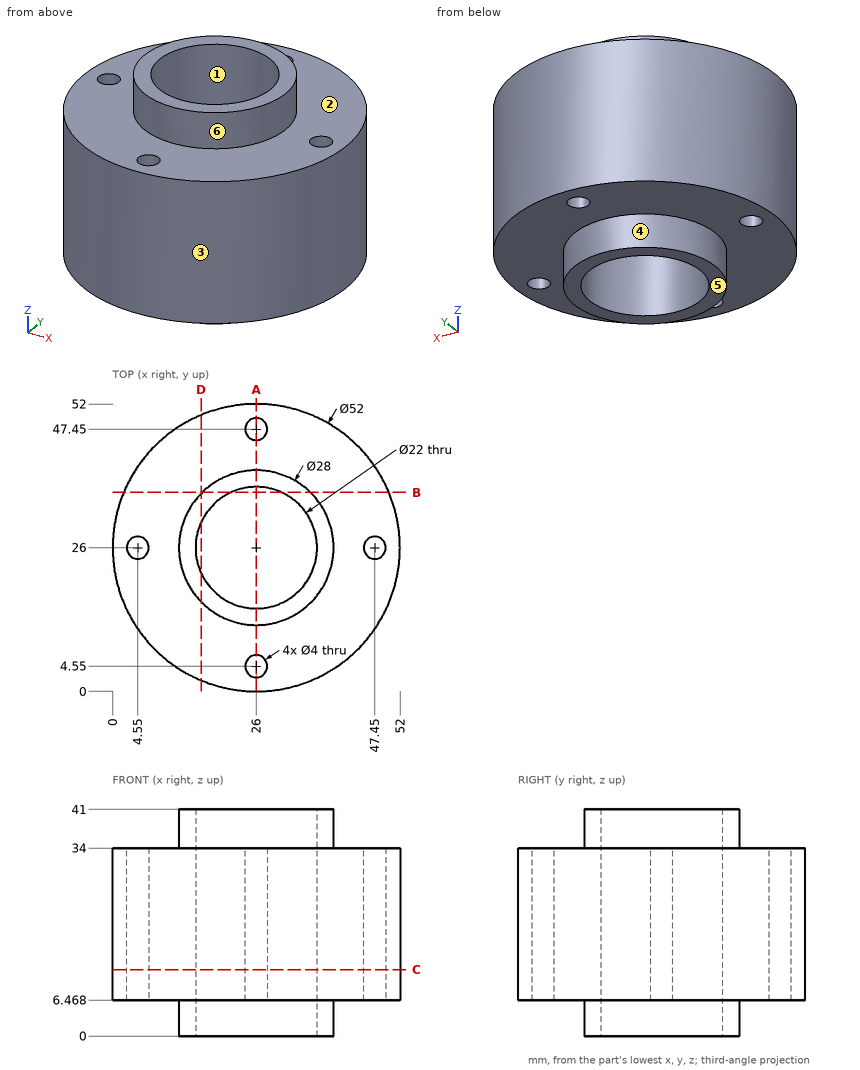
Study the drawing (mm; zero at the part's minimum x, y, z) and answer. A direction names the side the tool comes from. Give positions to 0.01 mm unless a question says otherwise; leave off trailing zeros. Order: outer loops, then holes, each group sorted by start corner. A loop starts at its lowest first (then second) coordinate and runs counter-clockwise, first axis right, second up.
1. Straight lines are drawn through the part: L1, parallel to Y at x = 26, z = 22; L2, parallel to Y at x = 26.5, z = 36; L3, parallel to Z at x = 13.5, y = 15.5. For each, find the intervals that lie inside material, in ascending order.
Result sheet:
L1: y = 0 to 2.55, 6.55 to 15, 37 to 45.45, 49.45 to 52
L2: y = 12.01 to 15.01, 36.99 to 39.99
L3: z = 6.47 to 34
2. Each of these flat-tipped pins is pushed along its axis until it touches: P1, Ø1.5, axis at x = 18, y = 6, coming from the -Z side; P2, Ø1.5, axis at y = 38, z = 14, coming from the +X side; P3, Ø1.5, axis at x = 16, y = 25, coming from the -Z side; P4, Ø5, axis at y = 26.5, z = 5, coming from the -X side. Where does it stop, or does it pass through?
Result sheet:
P1: stops at z = 6.47
P2: stops at x = 49.44
P3: passes through
P4: stops at x = 0
3. Section B-B, the plane y = 36 is taken. Determine the outline of the cut face in (x, z).
Result sheet:
outline: (2, 6.47) - (16.2, 6.47) - (16.2, 0) - (21.42, 0) - (21.42, 41) - (16.2, 41) - (16.2, 34) - (2, 34) - close; (30.58, 0) - (35.8, 0) - (35.8, 6.47) - (50, 6.47) - (50, 34) - (35.8, 34) - (35.8, 41) - (30.58, 41) - close
4. Section A-A, the plane x = 26 is taken. Determine the outline of the cut face in (y, z).
Result sheet:
outline: (0, 6.47) - (2.55, 6.47) - (2.55, 34) - (0, 34) - close; (6.55, 6.47) - (12, 6.47) - (12, 0) - (15, 0) - (15, 41) - (12, 41) - (12, 34) - (6.55, 34) - close; (37, 0) - (40, 0) - (40, 6.47) - (45.45, 6.47) - (45.45, 34) - (40, 34) - (40, 41) - (37, 41) - close; (49.45, 6.47) - (52, 6.47) - (52, 34) - (49.45, 34) - close
5. The mould has two halves that part along X. Classify the marked faces 1, 2 and 3: released by +X, released by -X, zero draft, split by the parting line, or undercut.
Result sheet:
face 1: undercut
face 2: zero draft
face 3: split by the parting line
6. For the marked faces 4, 5 and 6, determine the directions among +Z, -Z, +X, -X, +Y, -Y from which every point of the face is accessible in a straight line to the end or side of a thin tool.
Result sheet:
face 4: -Z
face 5: -Z, +X, -X, +Y, -Y
face 6: +Z
7. Section C-C, the plane z = 12 is taken. Determine the outline of the cut face in (x, y), and give its area (3 significant figures).
Result sheet:
outline: circle Ø52 at (26, 26); hole circle Ø4 at (4.55, 26); hole circle Ø22 at (26, 26); hole circle Ø4 at (26, 4.55); hole circle Ø4 at (26, 47.45); hole circle Ø4 at (47.45, 26)
area: 1,690 mm2
